from build123d import *

# Parameters (mm, degrees)
SKETCH_4_W           = 236
SKETCH_4_H           = 95
EXTRUDE_3_DEPTH      = 3
SKETCH_5_W           = 3
SKETCH_5_H           = 12.3
CUT_EXTRUDE_1_DEPTH  = 4
SKETCH_6_W           = 8
SKETCH_6_H           = 10.2
CUT_EXTRUDE_2_DEPTH  = 4
FILLET_2_R           = 1
FILLET_5_R           = 1
SKETCH_7_W           = 3
SKETCH_7_H           = 12.3
CUT_EXTRUDE_3_DEPTH  = 4
FILLET_6_R           = 1
SKETCH_8_W           = 8
SKETCH_8_H           = 10.2
CUT_EXTRUDE_5_DEPTH  = 4
FILLET_9_R           = 1
SKETCH_10_W          = 3
SKETCH_10_H          = 12.3
CUT_EXTRUDE_6_DEPTH  = 4
SKETCH_11_W          = 3
SKETCH_11_H          = 12.3
CUT_EXTRUDE_7_DEPTH  = 4
SKETCH_12_W          = 8
SKETCH_12_H          = 10.2
CUT_EXTRUDE_8_DEPTH  = 4
SKETCH_13_W          = 8
SKETCH_13_H          = 10.2
CUT_EXTRUDE_10_DEPTH = 4
FILLET_13_R          = 1
FILLET_15_R          = 1
FILLET_18_R          = 1
FILLET_19_R          = 1
SKETCH_14_R          = 1.5
SKETCH_14_R_2        = 2
SKETCH_14_R_3        = 2.5
CUT_EXTRUDE_11_DEPTH = 4
SKETCH_15_W          = 32
SKETCH_15_H          = 4
CUT_EXTRUDE_12_DEPTH = 4
FILLET_20_R          = 1


with BuildPart() as part:
    # 草图4 → 凸台-拉伸3 (new body)
    with BuildSketch(Plane(origin=(0, 0, 0), x_dir=(1, 0, 0), z_dir=(0, 1, 0))):
        Rectangle(SKETCH_4_W, SKETCH_4_H)
    extrude(amount=EXTRUDE_3_DEPTH)

    # 草图5 → 切除-拉伸1 (cut, through all)
    with BuildSketch(Plane(origin=(0, 3, 0), x_dir=(1, 0, 0), z_dir=(0, 1, 0))):
        with Locations((-116.5, 6.15)):
            Rectangle(SKETCH_5_W, SKETCH_5_H)
    extrude(amount=-CUT_EXTRUDE_1_DEPTH, mode=Mode.SUBTRACT)

    # 草图6 → 切除-拉伸2 (cut, through all)
    with BuildSketch(Plane(origin=(0, 3, 0), x_dir=(1, 0, 0), z_dir=(0, 1, 0))):
        with Locations((-114, 42.4)):
            Rectangle(SKETCH_6_W, SKETCH_6_H)
    extrude(amount=-CUT_EXTRUDE_2_DEPTH, mode=Mode.SUBTRACT)

    # 圆角2
    fillet_2_edges = [part.edges().sort_by_distance(p)[0] for p in [
        (-110, 1.5, -37.3),
    ]]
    fillet(fillet_2_edges, radius=FILLET_2_R)

    # 圆角5
    fillet_5_edges = [part.edges().sort_by_distance(p)[0] for p in [
        (-115, 1.5, -12.3),
    ]]
    fillet(fillet_5_edges, radius=FILLET_5_R)

    # 草图7 → 切除-拉伸3 (cut, through all)
    with BuildSketch(Plane(origin=(0, 3, 0), x_dir=(1, 0, 0), z_dir=(0, 1, 0))):
        with Locations((-116.5, -6.15)):
            Rectangle(SKETCH_7_W, SKETCH_7_H)
    extrude(amount=-CUT_EXTRUDE_3_DEPTH, mode=Mode.SUBTRACT)

    # 圆角6
    fillet_6_edges = [part.edges().sort_by_distance(p)[0] for p in [
        (-115, 1.5, 12.3),
    ]]
    fillet(fillet_6_edges, radius=FILLET_6_R)

    # 草图8 → 切除-拉伸5 (cut, through all)
    with BuildSketch(Plane(origin=(0, 3, 0), x_dir=(1, 0, 0), z_dir=(0, 1, 0))):
        with Locations((-114, -42.4)):
            Rectangle(SKETCH_8_W, SKETCH_8_H)
    extrude(amount=-CUT_EXTRUDE_5_DEPTH, mode=Mode.SUBTRACT)

    # 圆角9
    fillet_9_edges = [part.edges().sort_by_distance(p)[0] for p in [
        (-110, 1.5, 37.3),
    ]]
    fillet(fillet_9_edges, radius=FILLET_9_R)

    # 草图10 → 切除-拉伸6 (cut, through all)
    with BuildSketch(Plane(origin=(0, 3, 0), x_dir=(1, 0, 0), z_dir=(0, 1, 0))):
        with Locations((116.5, 6.15)):
            Rectangle(SKETCH_10_W, SKETCH_10_H)
    extrude(amount=-CUT_EXTRUDE_6_DEPTH, mode=Mode.SUBTRACT)

    # 草图11 → 切除-拉伸7 (cut, through all)
    with BuildSketch(Plane(origin=(0, 3, 0), x_dir=(1, 0, 0), z_dir=(0, 1, 0))):
        with Locations((116.5, -6.15)):
            Rectangle(SKETCH_11_W, SKETCH_11_H)
    extrude(amount=-CUT_EXTRUDE_7_DEPTH, mode=Mode.SUBTRACT)

    # 草图12 → 切除-拉伸8 (cut, through all)
    with BuildSketch(Plane(origin=(0, 3, 0), x_dir=(1, 0, 0), z_dir=(0, 1, 0))):
        with Locations((114, 42.4)):
            Rectangle(SKETCH_12_W, SKETCH_12_H)
    extrude(amount=-CUT_EXTRUDE_8_DEPTH, mode=Mode.SUBTRACT)

    # 草图13 → 切除-拉伸10 (cut, through all)
    with BuildSketch(Plane(origin=(0, 3, 0), x_dir=(1, 0, 0), z_dir=(0, 1, 0))):
        with Locations((114, -42.4)):
            Rectangle(SKETCH_13_W, SKETCH_13_H)
    extrude(amount=-CUT_EXTRUDE_10_DEPTH, mode=Mode.SUBTRACT)

    # 圆角13
    fillet_13_edges = [part.edges().sort_by_distance(p)[0] for p in [
        (110, 1.5, -37.3),
    ]]
    fillet(fillet_13_edges, radius=FILLET_13_R)

    # 圆角15
    fillet_15_edges = [part.edges().sort_by_distance(p)[0] for p in [
        (110, 1.5, 37.3),
    ]]
    fillet(fillet_15_edges, radius=FILLET_15_R)

    # 圆角18
    fillet_18_edges = [part.edges().sort_by_distance(p)[0] for p in [
        (115, 1.5, 12.3),
    ]]
    fillet(fillet_18_edges, radius=FILLET_18_R)

    # 圆角19
    fillet_19_edges = [part.edges().sort_by_distance(p)[0] for p in [
        (115, 1.5, -12.3),
    ]]
    fillet(fillet_19_edges, radius=FILLET_19_R)

    # 草图14 → 切除-拉伸11 (cut, through all)
    with BuildSketch(Plane(origin=(0, 3, 0), x_dir=(1, 0, 0), z_dir=(0, 1, 0))):
        with Locations((-106, 30.35)):
            Circle(SKETCH_14_R)
        with Locations((-28.28, 30.35)):
            Circle(SKETCH_14_R)
        with Locations((-106, 24.4)):
            Circle(SKETCH_14_R)
        with Locations((-48, 24.4)):
            Circle(SKETCH_14_R)
        with Locations((91.5, 6)):
            Circle(SKETCH_14_R_2)
        with Locations((91.5, 25)):
            Circle(SKETCH_14_R_2)
        with Locations((91.5, 36)):
            Circle(SKETCH_14_R_2)
        with Locations((69, 41.25)):
            Circle(SKETCH_14_R_3)
        with Locations((39, 16)):
            Circle(SKETCH_14_R_3)
        with Locations((19, 16)):
            Circle(SKETCH_14_R_3)
        with Locations((91.5, -6)):
            Circle(SKETCH_14_R_2)
        with Locations((91.5, -25)):
            Circle(SKETCH_14_R_2)
        with Locations((91.5, -36)):
            Circle(SKETCH_14_R_2)
        with Locations((69, -41.25)):
            Circle(SKETCH_14_R_3)
        with Locations((39, -16)):
            Circle(SKETCH_14_R_3)
        with Locations((19, -16)):
            Circle(SKETCH_14_R_3)
        with Locations((-28.28, -30.35)):
            Circle(SKETCH_14_R)
        with Locations((-48, -24.4)):
            Circle(SKETCH_14_R)
        with Locations((-106, -24.4)):
            Circle(SKETCH_14_R)
        with Locations((-106, -30.35)):
            Circle(SKETCH_14_R)
        with BuildLine():
            Line((-2.5, 24), (-2.5, -24))
            ThreePointArc((-2.5, -24), (-8.5, -30), (-14.5, -24))
            Line((-14.5, -24), (-14.5, 24))
            ThreePointArc((-14.5, 24), (-8.5, 30), (-2.5, 24))
        make_face()
        with BuildLine():
            Line((73, 26), (73, -26))
            ThreePointArc((73, -26), (69, -30), (65, -26))
            Line((65, -26), (65, 26))
            ThreePointArc((65, 26), (69, 30), (73, 26))
        make_face()
        with BuildLine():
            Line((-85.5, 32.85), (-67.5, 32.85))
            ThreePointArc((-67.5, 32.85), (-65, 30.35), (-67.5, 27.85))
            Line((-67.5, 27.85), (-85.5, 27.85))
            ThreePointArc((-85.5, 27.85), (-88, 30.35), (-85.5, 32.85))
        make_face()
        with BuildLine():
            Line((-85.5, -32.85), (-67.5, -32.85))
            ThreePointArc((-67.5, -32.85), (-65, -30.35), (-67.5, -27.85))
            Line((-67.5, -27.85), (-85.5, -27.85))
            ThreePointArc((-85.5, -27.85), (-88, -30.35), (-85.5, -32.85))
        make_face()
    extrude(amount=-CUT_EXTRUDE_11_DEPTH, mode=Mode.SUBTRACT)

    # 草图15 → 切除-拉伸12 (cut, through all)
    with BuildSketch(Plane(origin=(0, 3, 0), x_dir=(1, 0, 0), z_dir=(0, 1, 0))):
        with Locations((29, 47.5)):
            Rectangle(SKETCH_15_W, SKETCH_15_H)
        with Locations((29, -47.5)):
            Rectangle(SKETCH_15_W, SKETCH_15_H)
    extrude(amount=-CUT_EXTRUDE_12_DEPTH, mode=Mode.SUBTRACT)

    # 圆角20
    fillet_20_edges = [part.edges().sort_by_distance(p)[0] for p in [
        (13, 1.5, -45.5),
        (45, 1.5, -45.5),
        (45, 1.5, 45.5),
        (13, 1.5, 45.5),
    ]]
    fillet(fillet_20_edges, radius=FILLET_20_R)


solid = part.part
Here's how the part is built. I have some questions about the finished solid (model axes, mm). A direction names the side the tool comes from. Give positions to 0.01 mm unless a question says otherwise; leave off trailing zeros. Order: outer loops, then holes, each group sorted by start corner. A loop starts at its lowest first (then second) coordinate and runs counter-clockwise, first axis right, second up. Notation, with made-up numbers: M -33,16 L -19,16 A31 cw -19,47 Z; hole C -36,31.5 d2. An arc over 180 degrees is marked long. Answer as a JSON object with one key per item and string values. Group by question number.
1) Suppose I cut it at D-D, the plane z = 41.25. Write out the boundary of the cut face in (x, y).
2) Suppose I cut it at B-B, the plane x = -8.5. Write out the boundary of the cut face in (y, z).
3) I'm going to push flat-ended pins straight in: pin 1 Ø2.5 at (x, z) = (91.5, 36) entering from +Y; pin 2 Ø1 at (x, y) = (-116.5, 1.5) entering from -Z; pin 3 Ø1.5 at (x, y) = (33.5, 1) entering from +Z; pin 4 Ø0.8 at (y, z) = (1.5, 47) entering from -X. Where does each tip first touch, or does it pass through?
4) Suppose I cut it at C-C, the plane z = -16. Write out the boundary of the cut face in (x, y).
5) We'd pull the mould along X, two halves only. Please class faces 3 (the flat face through (-2, 0, -1)), 4 (the cylindrical face through (92.423, 1.521, -34.226)): pulls with the +X half, pulls with the -X half, needs draft (parallel to the pull), parting line crosses it, or undercut.
6) Please list where these lines run through material, in increasing order: L1, parallel to Z at x = 19, y = 1.1; L2, parallel to Z at x = -28.28, y = 1.7; L3, parallel to Z at x = -106, y = 1.6. Write a range as [from, to].
7) On a 3-axis mill with a long thin cutter (end or side, diameter ignored), from which of +Z, -Z, +X, -X, +Y, -Y can I reach the whole of each face in a straight line? I mean faces 1 (the flat face through (-2, 3, -1)), 2 (the cylindrical face through (-8.4, 1.5, 30)). Say none if no direction works.
8) Suppose I cut it at A-A, the plane x = -74. Write out the boundary of the cut face in (y, z).
Results found:
{
 "1": {"outline": "M -110,0 L 66.5,0 L 66.5,3 L -110,3 Z; M 71.5,0 L 110,0 L 110,3 L 71.5,3 Z"},
 "2": {"outline": "M 0,-47.5 L 3,-47.5 L 3,-30 L 0,-30 Z; M 0,30 L 3,30 L 3,47.5 L 0,47.5 Z"},
 "3": {"pin 1": "through", "pin 2": "z = -37.3", "pin 3": "z = 45.5", "pin 4": "x = -110"},
 "4": {"outline": "M -118,0 L -14.5,0 L -14.5,3 L -118,3 Z; M -2.5,0 L 16.5,0 L 16.5,3 L -2.5,3 Z; M 21.5,0 L 36.5,0 L 36.5,3 L 21.5,3 Z; M 41.5,0 L 65,0 L 65,3 L 41.5,3 Z; M 73,0 L 118,0 L 118,3 L 73,3 Z"},
 "5": {"face 3": "needs draft", "face 4": "undercut"},
 "6": {"L1": "[-45.5, -18.5], [-13.5, 13.5], [18.5, 45.5]", "L2": "[-47.5, -31.85], [-28.85, 28.85], [31.85, 47.5]", "L3": "[-47.5, -31.85], [-28.85, -25.9], [-22.9, 22.9], [25.9, 28.85], [31.85, 47.5]"},
 "7": {"face 1": "+Z, -Z, +X, -X, +Y", "face 2": "+Y, -Y"},
 "8": {"outline": "M 0,-47.5 L 3,-47.5 L 3,-32.85 L 0,-32.85 Z; M 0,-27.85 L 3,-27.85 L 3,27.85 L 0,27.85 Z; M 0,32.85 L 3,32.85 L 3,47.5 L 0,47.5 Z"}
}
